Input: part model. Units: mm. Frame: model coordinates. Round coordinates to 2 decimals unless told otherwise and drop trailing zeros. Answer as a JSON object with one key per item and string values.
```python
from build123d import *

# Parameters (mm, degrees)
SKETCH1_W           = 16.51
SKETCH1_H           = 22.225
BOSS_EXTRUDE1_DEPTH = 4.2926
FILLET1_R           = 2.54
SKETCH3_W           = 12.8778
SKETCH3_H           = 31.75
CUT_EXTRUDE1_DEPTH  = 4.2926
FILLET2_R           = 2.54
CUT_EXTRUDE2_DEPTH  = 4.2926


with BuildPart() as part:
    # Sketch1 → Boss-Extrude1 (new body)
    with BuildSketch(Plane.XY):
        with BuildLine():
            Line((-8.255, 171.081987477), (-8.255, 146.05))
            Line((-8.255, 146.05), (8.255, 146.05))
            Line((8.255, 146.05), (8.255, 42.644883355))
            add(Edge.make_bspline(
                [(125.716580007, 48.373759919), (101.454363005, 51.05167226), (61.670696801, 53.384876658), (22.758908367, 46.056998678), (8.255, 42.644883355)],
                knots=[0, 0, 0, 0, 0.621556192, 1, 1, 1, 1], degree=3))
            add(Edge.make_bspline(
                [(-8.255, 171.081987477), (8.482506786, 169.920834594), (37.696093446, 161.351973623), (91.678547842, 125.040727361), (116.930099327, 81.490043726), (125.716580007, 48.373759919)],
                knots=[0, 0, 0, 0, 0.260197261, 0.464601463, 1, 1, 1, 1], degree=3))
        make_face()
        Polygon((-8.255, 146.05), (-8.255, 22.225), (8.255, 22.225), (8.255, 42.644883355), (8.255, 146.05), align=None)
        with Locations((0, 11.1125)):
            Rectangle(SKETCH1_W, SKETCH1_H)
        Polygon((-16.891, 22.225), (-16.891, -22.225), (16.891, -22.225), (16.891, 22.225), (8.255, 22.225), (8.255, 0), (-8.255, 0), (-8.255, 22.225), align=None)
    extrude(amount=BOSS_EXTRUDE1_DEPTH)

    # Fillet1
    fillet1_edges = [part.edges().sort_by_distance(p)[0] for p in [
        (16.891, 22.225, 2.1463),
        (16.891, -22.225, 2.1463),
        (-16.891, -22.225, 2.1463),
        (-16.891, 22.225, 2.1463),
        (-8.255, 22.225, 2.1463),
        (8.255, 42.644883355, 2.1463),
        (8.255, 22.225, 2.1463),
    ]]
    fillet(fillet1_edges, radius=FILLET1_R)

    # Sketch3 → Cut-Extrude1 (cut)
    with BuildSketch(Plane.XY.offset(4.2926)):
        with Locations((0, -6.35)):
            Rectangle(SKETCH3_W, SKETCH3_H)
    extrude(amount=-CUT_EXTRUDE1_DEPTH, mode=Mode.SUBTRACT)

    # Fillet2
    fillet2_edges = [part.edges().sort_by_distance(p)[0] for p in [
        (6.4389, 9.525, 2.1463),
        (-6.4389, 9.525, 2.1463),
        (125.716580007, 48.373759919, 2.1463),
        (-8.255, 171.081987477, 2.1463),
    ]]
    fillet(fillet2_edges, radius=FILLET2_R)

    # Sketch4 → Cut-Extrude2 (cut)
    with BuildSketch(Plane(origin=(0, 0, 0), x_dir=(-1, 0, 0), z_dir=(0, 0, -1))):
        with BuildLine():
            Line((-9.622290965, 62.279587003), (-9.622290965, 137.454872526))
            add(Edge.make_bspline(
                [(-9.622290965, 137.454872526), (-31.976257123, 121.615669166), (-44.359940554, 97.193181134)],
                knots=[0, 0, 0, 1, 1, 1], degree=2))
            add(Edge.make_bspline(
                [(-44.359940554, 97.193181134), (-26.073912196, 80.643285354), (-9.622290965, 62.279587003)],
                knots=[0, 0, 0, 1, 1, 1], degree=2))
        make_face()
        with BuildLine():
            add(Edge.make_bspline(
                [(-65.171801242, 122.457122028), (-42.991307033, 146.419627916), (-9.622290965, 153.095219352)],
                knots=[0, 0, 0, 1, 1, 1], degree=2))
            add(Edge.make_bspline(
                [(-9.622290965, 153.095219352), (-36.425668846, 133.501984123), (-53.862303727, 105.466469115)],
                knots=[0, 0, 0, 1, 1, 1], degree=2))
            add(Edge.make_bspline(
                [(-65.171801242, 122.457122028), (-60.781840314, 113.076876159), (-53.862303727, 105.466469115)],
                knots=[0, 0, 0, 1, 1, 1], degree=2))
        make_face()
        with BuildLine():
            add(Edge.make_bspline(
                [(-72.704015401, 117.289439294), (-94.417782838, 93.472755404), (-98.988348102, 61.673623274)],
                knots=[0, 0, 0, 1, 1, 1], degree=2))
            add(Edge.make_bspline(
                [(-98.988348102, 61.673623274), (-82.698421223, 83.657662509), (-61.533499928, 100.794910417)],
                knots=[0, 0, 0, 1, 1, 1], degree=2))
            add(Edge.make_bspline(
                [(-72.704015401, 117.289439294), (-69.576013453, 107.271375671), (-61.533499928, 100.794910417)],
                knots=[0, 0, 0, 1, 1, 1], degree=2))
        make_face()
        with BuildLine():
            add(Edge.make_bspline(
                [(-86.321212925, 61.303058161), (-71.955525072, 78.774376711), (-53.329729843, 91.61675501)],
                knots=[0, 0, 0, 1, 1, 1], degree=2))
            add(Edge.make_bspline(
                [(-53.329729843, 91.61675501), (-36.084210617, 75.847325958), (-20.792276935, 58.171365413)],
                knots=[0, 0, 0, 1, 1, 1], degree=2))
            add(Edge.make_bspline(
                [(-86.321212925, 61.303058161), (-52.898087225, 72.583199638), (-20.792276935, 58.171365413)],
                knots=[0, 0, 0, 1, 1, 1], degree=2))
        make_face()
    extrude(amount=-CUT_EXTRUDE2_DEPTH, mode=Mode.SUBTRACT)


solid = part.part
```
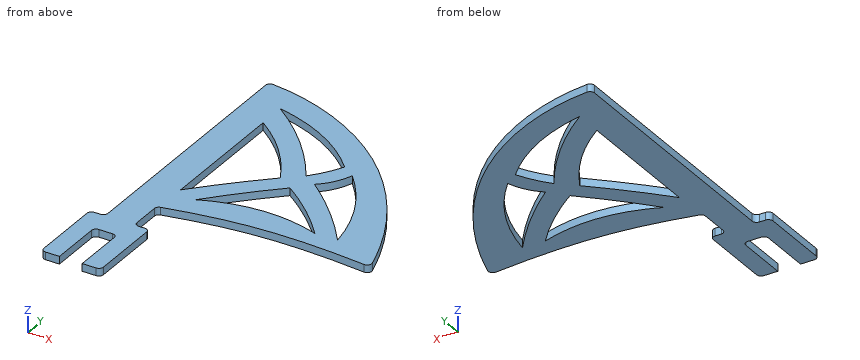
1) Section A-A, the plane z = 1.35. Count the separate pieces of the cut face and the enclosed holes in it, plus the area to 3 significant figures.
Output:
{"separate pieces": "1", "enclosed holes": "4", "area": "9,580 mm^2"}
2) Contact query for flat-ended pins moving along their axis: P1, Ø1, axis at x = 0.5, z = 3, coming from the +Y side; P2, Ø2, axis at y = 65, z = 2.5, coming from the -X side (3 decimals); P3, Ø1.3, axis at y = 32, z = 3, coming from the +X side (3 decimals). Output: stop coordinate, or through.
Output:
{"P1": "stops at y = 170.21", "P2": "stops at x = -8.255", "P3": "stops at x = 8.255"}
3) Ray query, probe 1 along Y at (x, z) = (69.5, 1.6); probe 2 along X at (y, z) = (81, 3.2) (3 decimals); probe 3 along X at (y, z) = (112.5, 2.7) (3 decimals). Return the intervals inside material, ascending.
Output:
{"probe 1": "y = 51.24 to 65.37, 78.88 to 94.02, 109.99 to 138.51", "probe 2": "x = -8.255 to 9.622, 27.341 to 42.159, 67.089 to 82.851, 94.379 to 113.687", "probe 3": "x = -8.255 to 9.622, 35.012 to 49.249, 59.457 to 70.832, 76.832 to 94.41"}
